Design review of the part built by this model. Coordinates are the model's own, in mm. Face numbers are marked on the shaded views. A direction names the side the tool comes from. Coordinates: 2 decimals unless noted, no trailing zeros. Write each loop counter-clockwise with the first axis right and the second up, starting at its lowest first coordinate (ties: lowest second). Pieces come first, ordered by that corner, then holes.
Q1. For pin 1 Ø1 at (x, z) = (-14.5, 25) entering from -Y; pin 2 Ø5.5 at (y, z) = (16.5, 1.5) entering from +X; pin 3 Ø5.5 at (y, z) = (19.5, 1.5) entering from -X, all flat-tipped, find the tip position at first contact; note any pin that passes through.
Q2. Take a section at C-C, the plane y = 21. Write out the cut boundary in (x, z), plus the area to 3 significant figures.
Q3. For L1, parallel to Z at x = -8, y = 34; L2, parallel to Z at x = 8.5, y = 34.15; L3, parallel to X at y = 34.85, z = 15, list the stretches that pass through material, from the lowest coordinate up.
Q4. Take a section at D-D, the plane z = 86.5. Write out the cut boundary in (x, y).
Q5. For the marked faces 1 and 2, list the 3-axis set-ups (+Z, -Z, +X, -X, +Y, -Y) from which the entire face can be reached by the end or side of a thin tool; tool diameter is ignored.
Q6. Take a section at B-B, the plane z = 15. Write out the cut boundary in (x, y).
Q7. Take a section at A-A, the plane x = 0. Write out the cut boundary in (y, z), plus the area to 4 significant figures.
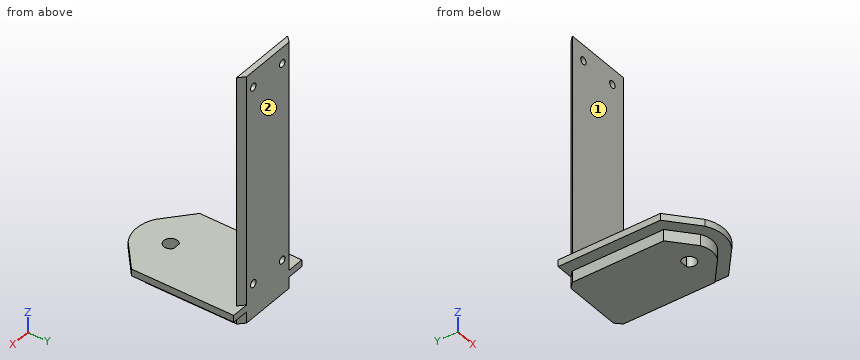
from build123d import *

# Parameters (mm, degrees)
BOSS_EXTRUDE1_DEPTH  = 8
BOSS_EXTRUDE3_DEPTH  = 109
M3_CLEARANCE_SLOT1_D = 3.2
BOSS_EXTRUDE4_DEPTH  = 3


with BuildPart() as part:
    # Sketch1 → Boss-Extrude1 (new body)
    with BuildSketch(Plane.XY):
        with BuildLine():
            Line((15, 33), (-15, 33))
            Line((-15, 33), (-15, -7))
            Line((-15, -7), (-5, -15.660254038))
            ThreePointArc((-5, -15.660254038), (0, -17), (5, -15.660254038))
            Line((5, -15.660254038), (15, -7))
            Line((15, -7), (15, 33))
        make_face()
        with BuildLine():
            Line((1.658312395, -4.5), (-1.658312395, -4.5))
            ThreePointArc((-1.658312395, -4.5), (0, -10), (1.658312395, -4.5))
        make_face(mode=Mode.SUBTRACT)
    extrude(amount=BOSS_EXTRUDE1_DEPTH)

    # Sketch1<5> → Boss-Extrude3 (add)
    with BuildSketch(Plane.XY):
        Polygon((-12.5, 35.5), (12.5, 35.5), (15, 33), (-15, 33), align=None)
    extrude(amount=BOSS_EXTRUDE3_DEPTH)

    # M3 Clearance Slot1 (through all)
    with Locations(Plane(origin=(0, 35.5, 0), x_dir=(1, 0, 0), z_dir=(0, 1, 0))):
        with Locations((-8.5, -15), (8.5, -15), (-8.5, -102), (8.5, -102)):
            Hole(M3_CLEARANCE_SLOT1_D / 2)

    # Sketch6 → Boss-Extrude4 (add)
    with BuildSketch(Plane.XY.offset(8)):
        with BuildLine():
            Line((-20, 35.5), (20, 35.5))
            Line((20, 35.5), (20, 33))
            Line((20, 33), (20, -9.284251259))
            Line((20, -9.284251259), (7.949555075, -19.720242691))
            ThreePointArc((7.949555075, -19.720242691), (0, -22), (-7.949555075, -19.720242691))
            Line((-7.949555075, -19.720242691), (-20, -9.284251259))
            Line((-20, -9.284251259), (-20, 33))
            Line((-20, 33), (-20, 35.5))
        make_face()
        with BuildLine():
            Line((1.658312395, -4.5), (-1.658312395, -4.5))
            ThreePointArc((-1.658312395, -4.5), (0, -10), (1.658312395, -4.5))
        make_face(mode=Mode.SUBTRACT)
    extrude(amount=-BOSS_EXTRUDE4_DEPTH)


solid = part.part
Responses:
1. pin 1: stops at y = 33
1. pin 2: stops at x = 15
1. pin 3: stops at x = -15
2. outline: (-20, 5) - (-15, 5) - (-15, 0) - (15, 0) - (15, 5) - (20, 5) - (20, 8) - (-20, 8) - close
2. area: 270 mm2
3. L1: z = 0 to 13.48, 16.52 to 100.48, 103.52 to 109
3. L2: z = 0 to 13.4, 16.6 to 100.4, 103.6 to 109
3. L3: x = -13.15 to -10.1, -6.9 to 6.9, 10.1 to 13.15
4. outline: (-15, 33) - (15, 33) - (12.5, 35.5) - (-12.5, 35.5) - close
5. face 1: +Z, +X, -X, -Y
5. face 2: +Z, -Z, +X, -X, +Y
6. outline: (-15, 33) - (-10.1, 33) - (-10.1, 35.5) - (-12.5, 35.5) - close; (-6.9, 33) - (6.9, 33) - (6.9, 35.5) - (-6.9, 35.5) - close; (10.1, 33) - (15, 33) - (12.5, 35.5) - (10.1, 35.5) - close
7. outline: (-22, 5) - (-17, 5) - (-17, 0) - (-10, 0) - (-10, 8) - (-22, 8) - close; (-4.5, 0) - (35.5, 0) - (35.5, 109) - (33, 109) - (33, 8) - (-4.5, 8) - close
7. area: 643.5 mm2
